Input: dimensioned drawing with shaded views. Units: mm. Origin: part minimum x, y, z. A direction names the side the tool comes from. Coordinates: 2 decimals unless noted, no trailing zeros. Order: outer loops, then holes, each group sorted by start corner. A loop starts at its lowest first (then second) coordinate and runs counter-clockwise, first axis right, second up. Notation, with made-up numbers: (63.25, 44) - (69.25, 44) arc R21 ccw to (69.25, 72) - close; hole circle Ø5 at (60, 52.5). An arc over 180 degrees is marked (long way). Use one line per item in the form item = value. Start each with the question number.
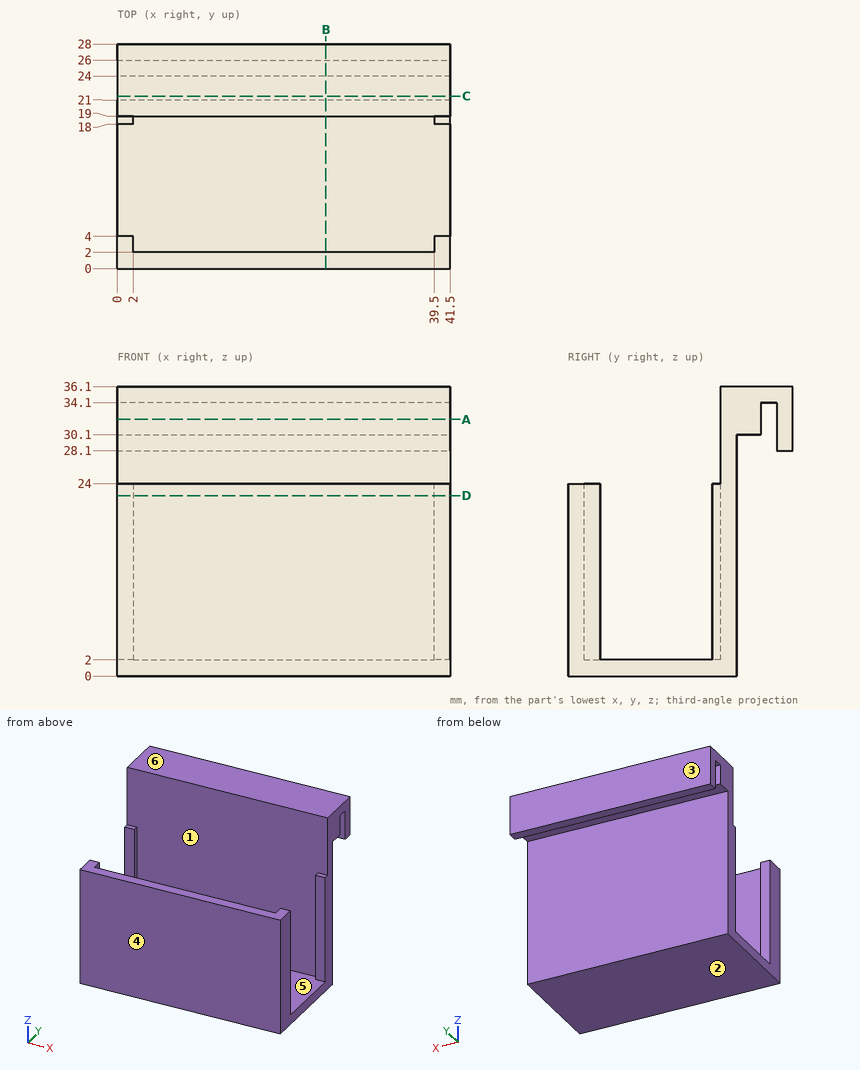
(1) Contact query for flat-ended pins moving along their axis: pin 1 Ø3 at (x, y) = (29.5, 1.5) entering from +Z; pin 2 Ø12 at (x, z) = (30.5, 10) entering from +Y; pin 3 Ø1.8 at (x, z) = (16, 31.5) entering from -Y; pin 4 Ø4 at (y, z) = (24.5, 16) entering from +X. Output: stop coordinate, or through.
(2) Cut plane B-B on x = 26. Return the cut outline in (y, z).
(3) Cut plane D-D on z = 22.5. Return the cut outline in (x, y), plus the area to 3 significant figures.
(4) Draft query along Y for the marked faces 3, 4, 5 and 6. Return one class per face: released by +Y, released by -Y, zero draft, split by the parting line, or undercut.
(5) Set-up query: the marked faces 1 and 2. Return all of +Z, -Z, +X, -X, +Y, -Y with unobstructed straight access to the full face (end or side cutting, diameter ignored); none if empty.
(6) Material intervals for L1, parallel to Y at x = 30, z = 7.5; L2, parallel to X at y = 2.75, z = 18; L3, parallel to Z at x = 7.5, y = 26.25, sorted ascending. Write a range as from..to.
(7) Cut plane C-C on y = 21.5. Return the cut outline in (x, z), plus the area to 3 significant figures.
(8) Cut plane A-A on z = 32. Return the cut outline in (x, y).
Check sheet entries:
q1.pin_1 = 24
q1.pin_2 = 21
q1.pin_3 = 19
q1.pin_4 = through
q2.outline = (0, 0) - (21, 0) - (21, 30.1) - (24, 30.1) - (24, 34.1) - (26, 34.1) - (26, 28.1) - (28, 28.1) - (28, 36.1) - (19, 36.1) - (19, 2) - (2, 2) - (2, 24) - (0, 24) - close
q3.outline = (0, 0) - (41.5, 0) - (41.5, 4) - (39.5, 4) - (39.5, 2) - (2, 2) - (2, 4) - (0, 4) - close; (0, 18) - (2, 18) - (2, 19) - (39.5, 19) - (39.5, 18) - (41.5, 18) - (41.5, 21) - (0, 21) - close
q3.area = 178 mm^2
q4.face_3 = released by +Y
q4.face_4 = released by -Y
q4.face_5 = undercut
q4.face_6 = zero draft
q5.face_1 = +Z
q5.face_2 = -Z, +X, -X, +Y, -Y
q6.L1 = 0..2, 19..21
q6.L2 = 0..2, 39.5..41.5
q6.L3 = 28.1..36.1
q7.outline = (0, 30.1) - (41.5, 30.1) - (41.5, 36.1) - (0, 36.1) - close
q7.area = 249 mm^2
q8.outline = (0, 19) - (41.5, 19) - (41.5, 24) - (0, 24) - close; (0, 26) - (41.5, 26) - (41.5, 28) - (0, 28) - close
